Could you check a few things on this model? Use its own coordinates, in mm. Face numbers are marked on the shaded views. A direction names the side the tool comes from. Round coordinates to 2 decimals unless told otherwise and drop trailing zeros. Loops run counter-clockwise (first coordinate to the right, second up) from the corner with the lowest first, then second, coordinate; pieces in that order, holes last. Notation, with made-up numbers: (68, 47) - (123, 47) arc R10 ccw to (123, 64) - close; hole circle Ø1 at (74, -25). An arc over 180 degrees is marked (long way). Use one line per item in the form item = value.
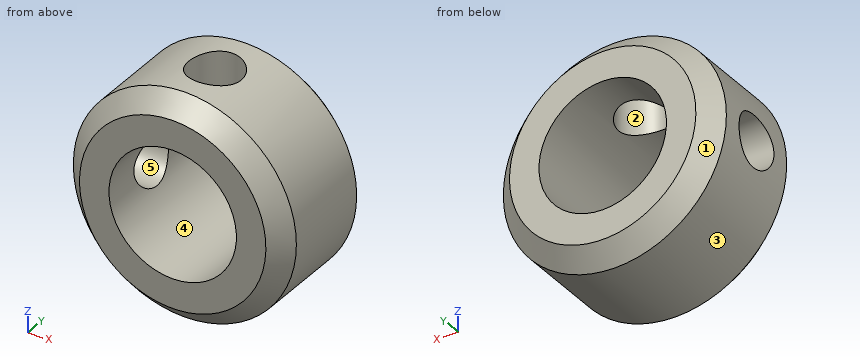
```python
from build123d import *

# Parameters (mm, degrees)
SKETCH1_R                  = 7
SKETCH1_R_2                = 4
BOSS_EXTRUDE1_DEPTH        = 4
M4X0_7_TAPPED_HOLE1_REACH  = 18.155
M4X0_7_TAPPED_HOLE1_BORE_R = 1.65
CHAMFER1_SIZE              = 1.15
CIRPATTERN1_COUNT          = 2
CIRPATTERN1_ANGLE          = 90


with BuildPart() as part:
    # Sketch1 → Boss-Extrude1 (new, symmetric)
    with BuildSketch(Plane(origin=(0, 0, 0), x_dir=(1, 0, 0), z_dir=(0, 1, 0))):
        with Locations(Location((0, 0, 0), (0, 0, 270))):
            Circle(SKETCH1_R)
        with Locations(Location((0, 0, 0), (0, 0, 270))):
            Circle(SKETCH1_R_2, mode=Mode.SUBTRACT)
    extrude(amount=BOSS_EXTRUDE1_DEPTH, both=True)

    # M4x0.7 Tapped Hole1 bore → M4x0.7 Tapped Hole1 (cut, up to next)
    with BuildSketch(Plane.XY.offset(7), mode=Mode.PRIVATE) as m4x0_7_tapped_hole1_sk1:
        Circle(M4X0_7_TAPPED_HOLE1_BORE_R)
    m4x0_7_tapped_hole1_tool1 = extrude(m4x0_7_tapped_hole1_sk1.sketch, amount=-M4X0_7_TAPPED_HOLE1_REACH, mode=Mode.PRIVATE) & part.part
    m4x0_7_tapped_hole1 = m4x0_7_tapped_hole1_tool1.solids().sort_by_distance((0, 0, 7))[0]
    add(m4x0_7_tapped_hole1, mode=Mode.SUBTRACT)

    # Chamfer1
    chamfer1_edges = [part.edges().sort_by_distance(p)[0] for p in [
        (0, -4, -7),
        (0, 4, -7),
    ]]
    chamfer(chamfer1_edges, length=CHAMFER1_SIZE)

    # CirPattern1: M4x0.7 Tapped Hole1 ×2 about axis
    cirpattern1_axis = Axis((0, 4, 0), (0, -1, 0))
    for i in range(1, CIRPATTERN1_COUNT):
        add(m4x0_7_tapped_hole1.rotate(cirpattern1_axis, i * CIRPATTERN1_ANGLE / (CIRPATTERN1_COUNT - 1)), mode=Mode.SUBTRACT)


solid = part.part
```
1. On a 3-axis mill with a long thin cutter (end or side, diameter ignored), from which of +Z, -Z, +X, -X, +Y, -Y can I reach the whole of each face in a straight line? I mean the marked faces 1 and 2. Say none if no direction works.
Solution:
face_1 = +Y
face_2 = +Z
2. If we section it at A-A, the plane z = 0: Write out the boundary of the cut face in (x, y), plus the area to 3 significant figures.
Solution:
outline = (-7, -2.85) - (-5.85, -4) - (-4, -4) - (-4, -1.65) - (-7, -1.65) - close; (-7, 1.65) - (-4, 1.65) - (-4, 4) - (-5.85, 4) - (-7, 2.85) - close; (4, -4) - (5.85, -4) - (7, -2.85) - (7, 2.85) - (5.85, 4) - (4, 4) - close
area = 35.5 mm^2
3. Please list where these lines run through material, in increasing order: line 1 along X through (y, z) = (1, 0); line 2 along Y through (x, z) = (-5.65, 0); line 3 along Z through (x, y) = (1.5, -1).
Solution:
line_1 = 4 to 7
line_2 = -4 to -1.65, 1.65 to 4
line_3 = -6.84 to -3.71, 3.71 to 6.84
4. We'd pull the mould along X, two halves only. Please class the marked faces 3, 4 and 5: +X half, -X half, draft (parallel to the pull), parting line (faces both ways), or undercut.
Solution:
face_3 = parting line
face_4 = undercut
face_5 = draft
5. For P1, Ø1.5, axis at x = 5, y = -2, coming from the +Z side, with a flat end and sliding along its axis, tell me the tip position at first contact or that it passes through.
Solution:
P1 = 5.56
6. If we section it at B-B, the plane x = 0: Write out the boundary of the cut face in (y, z).
Solution:
outline = (-4, -5.85) - (-2.85, -7) - (2.85, -7) - (4, -5.85) - (4, -4) - (-4, -4) - close; (-4, 4) - (-1.65, 4) - (-1.65, 7) - (-2.85, 7) - (-4, 5.85) - close; (1.65, 4) - (4, 4) - (4, 5.85) - (2.85, 7) - (1.65, 7) - close
